```python
from build123d import *

# Parameters (mm, degrees)
F0_W     = 100
F0_H     = 80
F0_R     = 15
F1_DEPTH = 25
F2_W     = 47.389767
F2_H     = 13.236273
F3_DEPTH = 50


with BuildPart() as f1:
    # F0 (on Top) → F1 (new body)
    with BuildSketch(Plane.XY):
        Rectangle(F0_W, F0_H)
        Circle(F0_R, mode=Mode.SUBTRACT)
    extrude(amount=F1_DEPTH)

    # F2 (on Right) → F3 (cut, symmetric)
    with BuildSketch(Plane.YZ):
        with Locations((-26.768697, 12.659147)):
            Rectangle(F2_W, F2_H)
    extrude(amount=F3_DEPTH, both=True, mode=Mode.SUBTRACT)


solid = f1.part
```
Here's how the part is built. I have some questions about the finished solid (model axes, mm). A direction names the side the tool comes from. Give positions to 0.01 mm unless a question says otherwise; leave off trailing zeros. Loops run counter-clockwise (first coordinate to the right, second up) from the corner with the lowest first, then second, coordinate; pieces in that order, holes last. Notation, with made-up numbers: M 33.5,13 L 73.5,13 A9 ccw 73.5,27 Z; hole C -29.75,76.5 d8. An arc over 180 degrees is marked long. Return JSON: item names as keys, results as strings.
Item 1: Imagine slicing it at A-A on y = 0. List the corners of the cut face in (x, z) for me.
A:
{"outline": "M -50,0 L -15,0 L -15,25 L -50,25 Z; M 15,0 L 50,0 L 50,25 L 15,25 Z"}
Item 2: Imagine slicing it at B-B on x = 0. List the corners of the cut face in (y, z) for me, then the cut area to 3 significant figures.
A:
{"outline": "M -40,0 L -15,0 L -15,6.04 L -40,6.04 Z; M -40,19.28 L -15,19.28 L -15,25 L -40,25 Z; M 15,0 L 40,0 L 40,25 L 15,25 Z", "area": "919 mm^2"}
Item 3: I'm going to push a flat-ended pin straight in: pin 1 Ø6.5 at (x, z) = (-25.5, 9.5) entering from -Y. Where does the tip first touch, or does it pass through?
A:
{"pin 1": "stops at y = -3.07"}
Item 4: Imagine slicing it at C-C on z = 4.75. List the corners of the cut face in (x, y) for me, then the cut area to 3 significant figures.
A:
{"outline": "M -50,-40 L 50,-40 L 50,40 L -50,40 Z; hole C 0,0 d30", "area": "7,290 mm^2"}
Item 5: Thinking about a two-plate mould opening in Z: for faces 1 (the flat face through (-1, 18, 0)), 2 (the flat face through (1, -22, 6.041)), 3 (the flat face through (-32, -3.074, 13)), 4 (the flat face through (-1, -40, 22)), which applies, released by +Z, released by -Z, zero draft, split by the parting line, or undercut?
A:
{"face 1": "released by -Z", "face 2": "undercut", "face 3": "undercut", "face 4": "zero draft"}
Item 6: On a 3-axis mill with a long thin cutter (end or side, diameter ignored), from which of +Z, -Z, +X, -X, +Y, -Y can I reach the whole of each face in a straight line? I mean faces 5 (the flat face through (50, 8, 12)), 6 (the flat face through (33, -3.074, 13)). Say none if no direction works.
A:
{"face 5": "+Z, -Z, +X, +Y, -Y", "face 6": "+X, -X, -Y"}
Item 7: Please list where these lines run through material, in increasing order: line 1 (Z direction, x = -42, y = -25.5); line 2 (Y direction, x = -35, z = 13); line 3 (Y direction, x = 0, z = 11.5).
A:
{"line 1": "z = 0 to 6.04, 19.28 to 25", "line 2": "y = -3.07 to 40", "line 3": "y = 15 to 40"}
Item 8: Imagine slicing it at D-D on x = -18.5. List the corners of the cut face in (y, z) for me.
A:
{"outline": "M -40,0 L 40,0 L 40,25 L -40,25 L -40,19.28 L -3.07,19.28 L -3.07,6.04 L -40,6.04 Z"}
